Verification items for the finished model (mm, model axes). A direction names the side the tool comes from. Coordinates: 2 decimals unless noted, no trailing zeros. Order: outer loops, then holes, each group sorted by start corner. A loop starts at its lowest first (then second) coordinate and runs counter-clockwise, first axis right, second up. Notation, with made-up numbers: (74.5, 51.25) -> (111.5, 51.25) arc R11 ccw to (111.5, 72.25) -> close; hole circle Ø8 at (86.5, 88). An arc over 180 degrees is marked (long way). Write item = value, one per line. Start each with the question number.
from build123d import *

# Parameters (mm, degrees)
F0_R     = 7
F1_DEPTH = 21.5
F2_R     = 5.5
F3_DEPTH = 43.001
F2_R_2   = 7
F4_DEPTH = 19
F6_R     = 5.5
F7_DEPTH = 12


with BuildPart() as f1:
    # F0 (on Front) → F1 (new body, symmetric)
    with BuildSketch(Plane.XZ):
        with BuildLine():
            Line((-14, 11), (-14, -7))
            Line((-14, -7), (-7, -14))
            Line((-7, -14), (21.0666262554, -14))
            ThreePointArc((21.0666262554, -14), (24.3318620364, -15.2134137678), (26.0122649968, -18.2647058824))
            ThreePointArc((26.0122649968, -18.2647058824), (28.3490951999, -26.115672061), (32.7880673968, -33))
            Line((32.7880673968, -33), (38, -33))
            Line((38, -33), (67, 0))
            Line((67, 0), (67, 19))
            Line((67, 19), (62, 24))
            Line((62, 24), (38, 24))
            ThreePointArc((38, 24), (29.5749729609, 16.2760691513), (18.2430849879, 14.7832519053))
            Line((18.2430849879, 14.7832519053), (0, 18))
            Line((0, 18), (-7, 18))
            Line((-7, 18), (-14, 11))
        make_face()
        Circle(F0_R, mode=Mode.SUBTRACT)
    extrude(amount=F1_DEPTH, both=True)

    # F2 (on face) → F3 (cut, through all)
    with BuildSketch(Plane.XZ.offset(21.5)):
        with Locations((53, 10)):
            Circle(F2_R)
    extrude(amount=-F3_DEPTH, mode=Mode.SUBTRACT)

    # F2 (on face) → F4 (cut)
    with BuildSketch(Plane.XZ.offset(21.5)):
        Polygon((15, -14), (15, 15.3550952894), (0, 18), (-7, 18), (-14, 11), (-14, -7), (-7, -14), align=None)
        Circle(F2_R_2, mode=Mode.SUBTRACT)
        with BuildLine():
            Line((54.696969697, -14), (21.0666262554, -14))
            ThreePointArc((21.0666262554, -14), (24.3318620364, -15.2134137678), (26.0122649968, -18.2647058824))
            ThreePointArc((26.0122649968, -18.2647058824), (28.3490951999, -26.115672061), (32.7880673968, -33))
            Line((32.7880673968, -33), (38, -33))
            Line((38, -33), (54.696969697, -14))
        make_face()
    extrude(amount=-F4_DEPTH, mode=Mode.SUBTRACT)

    # F6 (on offset) → F7 (cut, symmetric)
    with BuildSketch(Plane.XZ.offset(2.5)):
        with BuildLine():
            Line((67, 19), (62, 24))
            Line((62, 24), (38, 24))
            ThreePointArc((38, 24), (33.6653533969, 18.864697991), (27.8141459246, 15.5595718187))
            ThreePointArc((27.8141459246, 15.5595718187), (38.5714357733, -1.9228537457), (56.4545454545, -12))
            Line((56.4545454545, -12), (67, 0))
            Line((67, 0), (67, 19))
        make_face()
        with Locations((53, 10)):
            Circle(F6_R, mode=Mode.SUBTRACT)
    extrude(amount=F7_DEPTH, both=True, mode=Mode.SUBTRACT)


solid = f1.part
Item 1: Section check B-B (x = 53). Record the boundary of the cut face in (y, z), then the cut area to 3 significant figures.
Item 2: Section check A-A (y = 1.5). Record the boundary of the cut face in (x, z), then the cut area to 3 significant figures.
Item 3: Mould release check, pull along Y, two halves, no side actions. Record for faces 4 (the flat face through (-10, 9, 15)), 5 (the flat face through (47, -14.5, 10)), 6 (the flat face through (7, -2.5, 2)): pulls with the +Y half, pulls with the -Y half, needs draft (parallel to the pull), parting line crosses it, or undercut.
Item 4: Section check C-C (y = 17). Record the boundary of the cut face in (x, z), then the cut area to 3 significant figures.
Item 5: Section check D-D (z = -4.5). Record the boundary of the cut face in (x, y).
Item 6: Tool access check on faces 1 (the flat face through (15, -12, 0)), 2 (the flat face through (47, 9.5, 10)), 3 (the flat face through (38, -2.5, -21)). Record the directions out of +Z, -Z, +X, -X, +Y, -Y that give a thin tool (end or side, any length) a straight path to the whole face; none if there is none.
Item 7: Thickness scan on line 1 (Y direction, x = 36, z = 4.5); line 2 (Z direction, x = 53, y = -18); line 3 (Y direction, x = -1.5, z = -8). Record the ranges inside material, lowest first.
Item 8: Gauge pin test, flat ends, axial feed: P1, Ø5.5, axis at y = -15.5, z = -3, coming from the -X side; P2, Ø6, axis at x = 45.5, y = -3.5, coming from the -Z side; P3, Ø2, axis at x = -2.5, y = 4.5, coming from the +Z side; P4, Ø9, axis at x = 53, z = 10, coming from the +Y side. Record the tip position at first contact, or that the pin passes through.
Filled sheet:
q1.outline = (-21.5, -14) -> (-2.5, -14) -> (-2.5, -15.93) -> (21.5, -15.93) -> (21.5, 4.5) -> (9.5, 4.5) -> (9.5, -10.92) -> (-14.5, -10.92) -> (-14.5, 4.5) -> (-21.5, 4.5) -> close; (-21.5, 15.5) -> (-14.5, 15.5) -> (-14.5, 24) -> (-21.5, 24) -> close; (9.5, 15.5) -> (21.5, 15.5) -> (21.5, 24) -> (9.5, 24) -> close
q1.area = 633 mm^2
q2.outline = (-14, -7) -> (-7, -14) -> (21.07, -14) arc R5 cw to (26.01, -18.26) arc R29 ccw to (32.79, -33) -> (38, -33) -> (56.45, -12) arc R41 cw to (27.81, 15.56) arc R19 cw to (18.24, 14.78) -> (0, 18) -> (-7, 18) -> (-14, 11) -> close; hole circle Ø14 at (0, 0)
q2.area = 1,740 mm^2
q3.face_4 = needs draft
q3.face_5 = undercut
q3.face_6 = pulls with the -Y half
q4.outline = (-14, -7) -> (-7, -14) -> (21.07, -14) arc R5 cw to (26.01, -18.26) arc R29 ccw to (32.79, -33) -> (38, -33) -> (67, 0) -> (67, 19) -> (62, 24) -> (38, 24) arc R19 cw to (18.24, 14.78) -> (0, 18) -> (-7, 18) -> (-14, 11) -> close; hole circle Ø14 at (0, 0); hole circle Ø11 at (53, 10)
q4.area = 2,670 mm^2
q5.outline = (-14, -2.5) -> (-5.36, -2.5) -> (-5.36, 21.5) -> (-14, 21.5) -> close; (5.36, -2.5) -> (15, -2.5) -> (15, -21.5) -> (63.05, -21.5) -> (63.05, -14.5) -> (41.52, -14.5) -> (41.52, 9.5) -> (63.05, 9.5) -> (63.05, 21.5) -> (5.36, 21.5) -> close
q6.face_1 = +Z, -Z, -X, -Y
q6.face_2 = +Z, +X
q6.face_3 = -Z, +X, -X, -Y
q7.line_1 = -21.5 to -14.5, 9.5 to 21.5
q7.line_2 = -14 to 4.5, 15.5 to 24
q7.line_3 = -2.5 to 21.5
q8.P1 = 15
q8.P2 = -27.68
q8.P3 = 18
q8.P4 = through
